Drawing for the job (mm, zero at the part's lowest x, y, z). Give positions to 0.01 mm unless a question says otherwise; leave off trailing zeros. Write each loop counter-clockwise with the first axis right and the second up, starting at its lowest first coordinate (ties: lowest second). Pieces come first, ordered by that corner, then holes. Notation, with made-up numbers: M 26.5,72 L 75.5,72 A18 ccw 75.5,85 Z; hole C -10,-25.75 d9. An arc over 180 degrees is marked long. Write item = value, one per line. Start each with the question number.
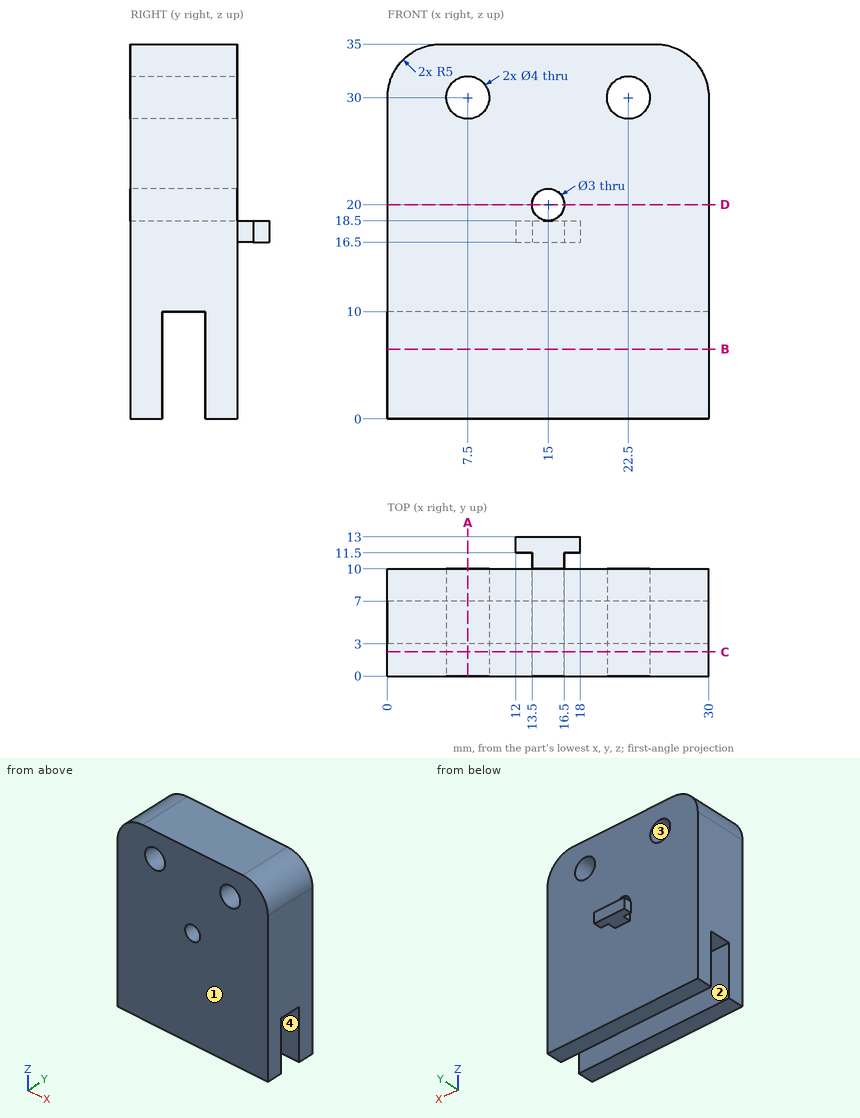
Q1. Drop flat-ended pins along their axis: P1, Ø3, axis at x = 21, z = 7, coming from the -Y side; P2, Ø1.5, axis at x = 16, y = 11.5, coming from the -Z side; P3, Ø6.5, axis at x = 7.5, z = 30, coming from the +Y side; P4, Ø3, axis at x = 16.5, y = 5, coming from the -Z side. Give the stop position or say it passes through.
Q2. Probe line 1 along X through (y, z) = (5.75, 30); line 2 along X through (y, z) = (8, 20); line 3 along Y through (x, z) = (20.75, 9). List the from-to ranges inside material, lowest first.
Q3. Slice it at A-A (x = 7.5). Give the cut face in (y, z), and give its area (3 significant figures).
Q4. Two-plate mould, pull along Y, no slides. Class the marked faces 1, 2, 3 and 4: +Y half, -Y half, draft (parallel to the pull), parting line (faces both ways), or undercut.
Q5. Slice it at B-B (z = 6.5). Give the cut face in (x, y).
Q6. Slice it at C-C (y = 2.25). Give the cut face in (x, z).
Q7. Slice it at D-D (z = 20). Give the cut face in (x, y).
Working result:
q1.P1 = 0
q1.P2 = 16.5
q1.P3 = 10
q1.P4 = 10
q2.line_1 = 0 to 5.5, 9.5 to 20.5, 24.5 to 30
q2.line_2 = 0 to 13.5, 16.5 to 30
q2.line_3 = 0 to 3, 7 to 10
q3.outline = M 0,0 L 3,0 L 3,10 L 7,10 L 7,0 L 10,0 L 10,28 L 0,28 Z; M 0,32 L 10,32 L 10,35 L 0,35 Z
q3.area = 270 mm2
q4.face_1 = -Y half
q4.face_2 = undercut
q4.face_3 = draft
q4.face_4 = undercut
q5.outline = M 0,0 L 30,0 L 30,3 L 0,3 Z; M 0,7 L 30,7 L 30,10 L 0,10 Z
q6.outline = M 0,0 L 30,0 L 30,30 A5 ccw 25,35 L 5,35 A5 ccw 0,30 Z; hole C 7.5,30 d4; hole C 15,20 d3; hole C 22.5,30 d4
q7.outline = M 0,0 L 13.5,0 L 13.5,10 L 0,10 Z; M 16.5,0 L 30,0 L 30,10 L 16.5,10 Z
